```python
from build123d import *

# Parameters (mm, degrees)
SKETCH1_W                       = 20
SKETCH1_H                       = 46.45
BOSS_EXTRUDE1_DEPTH             = 5
BOSS_EXTRUDE4_REACH             = 27.776
BOSS_EXTRUDE4_DIRECTION_2_REACH = 27.776
SKETCH6_R                       = 1.45
CUT_EXTRUDE2_DEPTH              = 7.5


with BuildPart() as part:
    # Sketch1 → Boss-Extrude1 (new body)
    with BuildSketch(Plane.XY):
        Rectangle(SKETCH1_W, SKETCH1_H)
    extrude(amount=BOSS_EXTRUDE1_DEPTH)

    # Boss-Extrude4: up to this face of the body (flat: up to its plane)
    boss_extrude4_end = Plane(part.part.faces().sort_by_distance((0, 23.225, 2.5))[0])
    # Sketch4 → Boss-Extrude4 (add, up to the picked face)
    with BuildSketch(Plane(origin=(0, 0, 0), x_dir=(1, 0, 0), z_dir=(0, 1, 0)), mode=Mode.PRIVATE) as boss_extrude4_sk1:
        Polygon((3.55, -5), (-16.45, -5), (-16.45, 25), (10, 0), (10, -5), align=None)
    boss_extrude4_tool1 = split(extrude(boss_extrude4_sk1.sketch, amount=BOSS_EXTRUDE4_REACH, mode=Mode.PRIVATE), bisect_by=boss_extrude4_end, keep=Keep.BOTH, mode=Mode.PRIVATE)
    add(boss_extrude4_tool1.solids().sort_by(Axis((-6.37381, 0, -5.238095), (0, 1, 0)))[0])

    # Boss-Extrude4 direction 2: up to this face of the body (flat: up to its plane)
    boss_extrude4_direction_2_end = Plane(part.part.faces().sort_by_distance((0, -23.225, 2.5))[0])
    # Sketch4 → Boss-Extrude4 direction 2 (add, up to the picked face)
    with BuildSketch(Plane(origin=(0, 0, 0), x_dir=(1, 0, 0), z_dir=(0, 1, 0)), mode=Mode.PRIVATE) as boss_extrude4_direction_2_sk1:
        Polygon((3.55, -5), (-16.45, -5), (-16.45, 25), (10, 0), (10, -5), align=None)
    boss_extrude4_direction_2_tool1 = split(extrude(boss_extrude4_direction_2_sk1.sketch, amount=-BOSS_EXTRUDE4_DIRECTION_2_REACH, mode=Mode.PRIVATE), bisect_by=boss_extrude4_direction_2_end, keep=Keep.BOTH, mode=Mode.PRIVATE)
    add(boss_extrude4_direction_2_tool1.solids().sort_by(Axis((-6.37381, 0, -5.238095), (0, -1, 0)))[0])

    # Sketch6 → Cut-Extrude2 (cut)
    with BuildSketch(Plane.XY.offset(5)):
        with Locations((3.55, 16.775)):
            Circle(SKETCH6_R)
        with Locations((3.55, 1.935)):
            Circle(SKETCH6_R)
    extrude(amount=-CUT_EXTRUDE2_DEPTH, mode=Mode.SUBTRACT)


solid = part.part
```
Check sheet for the modelled part. Datum: model origin and axes. Units: mm. A direction names the side the tool comes from. Round coordinates to 2 decimals unless told otherwise and drop trailing zeros. Order: outer loops, then holes, each group sorted by start corner. A loop starts at its lowest first (then second) coordinate and runs counter-clockwise, first axis right, second up. Notation, with made-up numbers: (81, -28) -> (119, -28) arc R18 ccw to (119, -18) -> close; hole circle Ø10 at (56, 32.25). An arc over 180 degrees is marked (long way). One line per item, written item: value. Start each with the question number.
Q1. Cross-section at D-D (z = -14). Record the boundary of the cut face in (x, y) (3 decimals), and give its area (3 significant figures).
Q2. Thickness scan on line 1 (Y direction, x = 3.55, z = 2.75) (3 decimals); line 2 (X direction, y = -16, z = -3); line 3 (Z direction, x = -8, y = -2.5). Record the ranges inside material, lowest first.
Q3. Cross-section at B-B (x = 3.55). Record the boundary of the cut face in (y, z) (3 decimals).
Q4. Cross-section at A-A (y = 8). Record the boundary of the cut face in (x, z), and give its area (3 significant figures).
Q5. Cross-section at C-C (z = -0.5). Record the boundary of the cut face in (x, y) (3 decimals).
Q6. Gauge pin test, flat ends, axial feed: pin 1 Ø3.5 at (x, y) = (3.55, 16.775) entering from -Z; pin 2 Ø12 at (y, z) = (-1.5, -16.5) entering from +X; pin 3 Ø8 at (x, y) = (-9.5, -5.5) entering from -Z. Record the tip position at first contact, or that the pin passes through.
Q7. Mould release check, pull along Y, two halves, no side actions. Record for faces 3 (the face through (4, 2, -2.5)), 4 (the face through (2.481, 2.915, 1.303)), 5 (the face through (-16.45, 0, -10)), 6 (the face through (-6, -23.225, -6)): pulls with the +Y half, pulls with the -Y half, needs draft (parallel to the pull), parting line crosses it, or undercut.
Q8. Set-up check for faces 1 (the face through (4, 17, -2.5)), 2 (the face through (-6, 23.225, -7)): record each of +Z, -Z, +X, -X, +Y, -Y from which the full face is reachable in a straight line by a thin tool's end or side.
Completed:
1. outline: (-16.45, -23.225) -> (-4.812, -23.225) -> (-4.812, 23.225) -> (-16.45, 23.225) -> close
1. area: 541 mm²
2. line 1: y = -23.225 to 0.485, 3.385 to 15.325, 18.225 to 23.225
2. line 2: x = -16.45 to 6.83
2. line 3: z = -17.01 to 5
3. outline: (-23.225, -6.096) -> (23.225, -6.096) -> (23.225, 5) -> (18.225, 5) -> (18.225, -2.5) -> (15.325, -2.5) -> (15.325, 5) -> (3.385, 5) -> (3.385, -2.5) -> (0.485, -2.5) -> (0.485, 5) -> (-23.225, 5) -> close
4. outline: (-16.45, -25) -> (10, 0) -> (10, 5) -> (-16.45, 5) -> close
4. area: 463 mm²
5. outline: (-16.45, -23.225) -> (9.471, -23.225) -> (9.471, 23.225) -> (-16.45, 23.225) -> close; hole circle Ø2.9 at (3.55, 1.935); hole circle Ø2.9 at (3.55, 16.775)
6. pin 1: stops at z = -7.75
6. pin 2: stops at x = -1.11
6. pin 3: stops at z = -22.21
7. face 3: undercut
7. face 4: undercut
7. face 5: needs draft
7. face 6: pulls with the -Y half
8. face 1: +Z
8. face 2: +Z, -Z, +X, -X, +Y
